Autodesk Inventor part; units mm, degrees
ref_plane "Work Plane1" through (30.1625, 0, 0) normal (0, 0, -1) x (1, 0, 0)
ref_plane "YZ Plane" through (0, 0, 0) normal (1, 0, 0) x (0, 1, 0)
ref_plane "XZ Plane" through (0, 0, 0) normal (0, 1, 0) x (-1, 0, 0)
sketch "Sketch1" plane through (0, 0, 0) normal (0, 0, 1) x (1, 0, 0)
  line L0 (-3.3, 0) -> (25, 0)
  line L1 (25, 0) -> (25, 2.5)
  line L2 (25, 2.5) -> (1.6, 2.5)
  line L3 (1.6, 2.5) -> (1.1091, 2.2547)
  line L4 (1.1091, 2.2547) -> (0, 2.2547)
  line L5 (0, 2.2547) -> (0, 4.25)
  line L6 (-8.96, 0) -> (30.66, 0)
  line L7 (0, -0.85) -> (0, 5.1)
  line L8 (-3.3, 0) -> (-3.3, 3.9613)
  line L9 (0, 4.25) -> (-3.3, 3.9613)
  line L10 (1.6, 2.5) -> (0, 2.5) construction
  dimension "d0" = 25
  dimension "d1" = 23.4
  dimension "d2" = 0.4909
  dimension "d3" = 3.3
  dimension "d4" = 5
  dimension "d5" = 4.5095
  dimension "d9" = 8.5
  dimension "d10" = 5
revolve "Body" add sketch "Sketch1" angle 360 about axis through (-3.3, 0, 0) along (1, 0, 0)
sketch "Sketch2" plane through (-3.3, 0, 0) normal (-1, 0, 0) x (0, 0, 1)
  circle A0 centre (0, 0) radius 4.25
  line L0 (0, 0) -> (0, 3.9613)
  line L1 (-4.25, 0.6) -> (4.25, 0.6)
  line L2 (4.25, 0.6) -> (4.25, -0.6)
  line L3 (4.25, -0.6) -> (-4.25, -0.6)
  line L4 (-4.25, -0.6) -> (-4.25, 0.6)
  line L5 (-4.25, 0) -> (4.25, 0) construction
  line L6 (0, 0.6) -> (0, -0.6) construction
  point P0 (0, 0)
  dimension "d11" = 1.2
  dimension "d12" = 8.5
fillet "Fillet1" radius 0.2 1 edges at (-3.3, -3.9613, 0)
extrude "Slot" cut sketch "Sketch2" against normal blind 1.3 contours A0 L3 L1 | L2 L3 A0 | A0 L1 L2 | A0 L4 L1 | L3 L4 A0
thread "Thread"
chamfer "Chamfer1" distance 0.4908 distance2 0.4909 1 edges at (25, -2.5, 0) measured on face at (25, 0.6238, 0.5526)
ref_plane "Work Plane1" through (30.1625, 0, 0) normal (0, 0, -1) x (1, 0, 0)
equation "\"d11\" = SBR"
equation "\"d12\" = KOD"
equation "\"d19\" = STI"
equation "\"d14\" = RR"
equation "\"d15\" = GEL"
equation "\"d17\" = -0.5 * SPD + 0.5 * GD"
equation "\"d0\" = NLG"
equation "\"d1\" = GEL"
equation "\"d3\" = KOH"
equation "\"d4\" = GD"
equation "\"d5\" = BDM"
equation "\"d9\" = KOD"
equation "\"d10\" = KEWI"
equation "\"GD\" = NND"
equation "\"NLG\" = 25"
equation "\"GEL\" = 23.4"
equation "\"KOD\" = 8.5"
equation "\"KOH\" = 3.3"
equation "\"GAL\" = 0.61345 * PTC"
equation "\"SPD\" = NND - 1.2269 * PTC"
equation "\"BDM\" = 4.5095"
equation "\"GUL\" = 0.61345 * PTC"
equation "\"RR\" = 0.2"
equation "\"SBR\" = 1.2"
equation "\"STI\" = 1.3"
equation "\"KEWI\" = 5deg"
equation "\"PTC\" = 0.8"
equation "\"THREADDIA\" = 5"
equation "\"TOA\" = 30deg"
equation "\"NND\" = 5"
equation "\"GD1\" = THREADDIA - 1.2269 * PTC"
properties part number "ISO 1207 - M5 x 25" material "Stainless Steel, 440C"
Work out the finished part from the listing and answer in its coordinate system (mm). A direction names the side the tool comes from. Coordinates: 2 decimals unless noted, no trailing zeros. Loops run counter-clockwise (first coordinate to the right, second up) from the corner with the lowest first, then second, coordinate; pieces in that order, holes last. Notation, with made-up numbers: (-23.5, 45) -> (10.5, 45) arc R30 ccw to (10.5, 82) -> close; hole circle Ø10 at (32, 34.5). An arc over 180 degrees is marked (long way). Answer as CSV lines item,"result".
Q1. Each of these flat-tipped pins is pushed along its axis until it touches: pin 1 (1.5 mm diameter, centred on x = 6.5, z = -1.5, fed in from -Y); pin 2 (1.5 mm diameter, centred on y = 3, z = -2, fed in from +X); pin 3 (4 mm diameter, centred on x = 13.5, z = -1, fed in from +Y). Where does it stop, or does it pass through?
Findings:
pin 1,"stops at y = -2.38"
pin 2,"stops at x = 0"
pin 3,"stops at y = 2.5"
Q2. For a pull along Y with two mould halves and no side action, classify faces 1 (the face through (-2, 0, 0)), 2 (the face through (12.89, -0.54, 2.44)), 3 (the face through (0, 2, -2)), 4 (the face through (-3, -0.6, 0)) as +Y half, -Y half, draft (parallel to the pull), parting line (faces both ways), or undercut.
Findings:
face 1,"undercut"
face 2,"parting line"
face 3,"draft"
face 4,"undercut"
Q3. The part is cut by section A-A on y = 0. Write down the section's boundary in (x, z).
Findings:
outline,"(-2, -4.08) -> (0, -4.25) -> (0, -2.25) -> (1.11, -2.25) -> (1.6, -2.5) -> (24.51, -2.5) -> (25, -2.01) -> (25, 2.01) -> (24.51, 2.5) -> (1.6, 2.5) -> (1.11, 2.25) -> (0, 2.25) -> (0, 4.25) -> (-2, 4.08) -> close"
Q4. A tool of negligible diameter and unlimited length cuts with its end or side. For faces 5 (the face through (-3, 0.6, 0)), 6 (the face through (0.55, -1.79, 1.37)), 7 (the face through (-3.3, 2, 0)), from which of +Z, -Z, +X, -X, +Y, -Y can it reach the whole face along a straight path? Write none if from no direction.
Findings:
face 5,"+Z, -Z, -X"
face 6,"none"
face 7,"+Z, -Z, -X, +Y, -Y"
Q5. The part is cut by section C-C on x = 3.25. Write down the section's boundary in (y, z).
Findings:
outline,"circle Ø5 at (0, 0)"
Q6. The part is cut by section B-B on z = 0. Write down the section's boundary in (x, y).
Findings:
outline,"(-3.3, -3.78) arc R0.2 ccw to (-3.12, -3.98) -> (0, -4.25) -> (0, -2.25) -> (1.11, -2.25) -> (1.6, -2.5) -> (24.51, -2.5) -> (25, -2.01) -> (25, 2.01) -> (24.51, 2.5) -> (1.6, 2.5) -> (1.11, 2.25) -> (0, 2.25) -> (0, 4.25) -> (-3.12, 3.98) arc R0.2 ccw to (-3.3, 3.78) -> (-3.3, 0.6) -> (-2, 0.6) -> (-2, -0.6) -> (-3.3, -0.6) -> close"
Q7. Find the intervals of material crossed by probe 1 along X at (y, z) = (3.5, 1.5); probe 2 along X at (y, z) = (1, -1.75); probe 3 along Z at (x, y) = (0.5, 0.25), in increasing order.
Findings:
probe 1,"x = -3.3 to 0"
probe 2,"x = -3.3 to 24.99"
probe 3,"z = -2.24 to 2.24"
